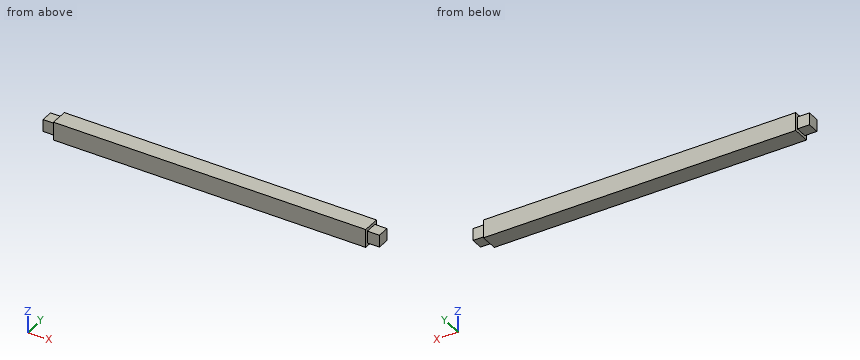
```python
from build123d import *

# Parameters (mm, degrees)
F0_W     = 1290
F0_H     = 75
F1_DEPTH = 72
F2_W     = 50
F2_H     = 50
F3_DEPTH = 50
F4_W     = 50
F4_H     = 50
F5_DEPTH = 50


with BuildPart() as f1:
    # F0 (on Front) → F1 (new body)
    with BuildSketch(Plane.XZ):
        with Locations((498.112862, 5.05404)):
            Rectangle(F0_W, F0_H)
    extrude(amount=F1_DEPTH)

    # F2 (on face) → F3 (join)
    with BuildSketch(Plane.YZ.offset(1143.112862)):
        with Locations((-36, 5.05404)):
            Rectangle(F2_W, F2_H)
    extrude(amount=F3_DEPTH)

    # F4 (on face) → F5 (join)
    with BuildSketch(Plane(origin=(-146.887138, 0, 0), x_dir=(0, -1, 0), z_dir=(-1, 0, 0))):
        with Locations((36, 5.05404)):
            Rectangle(F4_W, F4_H)
    extrude(amount=F5_DEPTH)


solid = f1.part
```
The listing builds one solid part. Answer for the finished solid, in the listing's coordinates (mm). Coordinates: 2 decimals unless noted, no trailing zeros. Write each loop counter-clockwise with the first axis right and the second up, starting at its lowest first coordinate (ties: lowest second). Pieces come first, ordered by that corner, then holes. Notation, with made-up numbers: (44, -26.75) - (76, -26.75) arc R22 ccw to (76, -6.75) - close; hole circle Ø6 at (31, -31). An arc over 180 degrees is marked (long way). Return JSON: item names as keys, results as strings. Group by question number.
Q1. Find the intervals of material crossed by line 1 along X through (y, z) = (-26, 38.5), in increasing order. Write a range as [from, to].
Q2. The part is cut by section A-A on z = 3.5. Write down the section's boundary in (x, y).
Q3. The part is cut by section B-B on y = -48.5. Write down the section's boundary in (x, z).
Q4. Flat-ended cylindrical pins translate along their axes: pin 1 Ø15 at (x, y) = (-172.5, -46.5) entering from +Z; pin 2 Ø25 at (x, y) = (-172.5, -34) entering from -Z; pin 3 Ø25 at (x, z) = (1178.5, 11) entering from +Y. Find the tip coordinate at first contact, or state that the pin passes through.
Evaluation:
{
 "1": {"line 1": "x = [-146.89, 1143.11]"},
 "2": {"outline": "(-196.89, -61) - (-146.89, -61) - (-146.89, -72) - (1143.11, -72) - (1143.11, -61) - (1193.11, -61) - (1193.11, -11) - (1143.11, -11) - (1143.11, 0) - (-146.89, 0) - (-146.89, -11) - (-196.89, -11) - close"},
 "3": {"outline": "(-196.89, -19.95) - (-146.89, -19.95) - (-146.89, -32.45) - (1143.11, -32.45) - (1143.11, -19.95) - (1193.11, -19.95) - (1193.11, 30.05) - (1143.11, 30.05) - (1143.11, 42.55) - (-146.89, 42.55) - (-146.89, 30.05) - (-196.89, 30.05) - close"},
 "4": {"pin 1": "stops at z = 30.05", "pin 2": "stops at z = -19.95", "pin 3": "stops at y = -11"}
}
